```python
from build123d import *

# Parameters (mm, degrees)
SHELL1_T            = -1
SKETCH2_R           = 45
SKETCH2_R_2         = 3.125
SKETCH2_R_3         = 28.999861121
BOSS_EXTRUDE1_DEPTH = 2


with BuildPart() as part:
    # Sketch1 → Revolve1 (revolve)
    with BuildSketch(Plane(origin=(0, 0, 0), x_dir=(0, 0, -1), z_dir=(1, 0, 0))):
        with BuildLine():
            Line((0, 0), (-50.959835356, 0))
            Line((-50.959835356, 0), (-60.054255014, 0))
            Line((-60.054255014, 0), (-60.054255014, 30))
            Line((-60.054255014, 30), (-30.054255014, 29.5))
            ThreePointArc((-30.054255014, 29.5), (-27.754838856, 29.797720054), (-25.637373582, 30.742332522))
            ThreePointArc((-25.637373582, 30.742332522), (-22.902920152, 32.314145749), (-20.042663952, 33.643343571))
            ThreePointArc((-20.042663952, 33.643343571), (-10.179122164, 36.1760026), (0, 35.877187771))
            Line((0, 35.877187771), (0, 34.862194457))
            Line((0, 34.862194457), (0, 0))
        make_face()
    revolve(axis=Axis((0, 0, 0), (0, 0, 1)))

    # Shell1
    shell1_openings = [part.faces().sort_by_distance(p)[0] for p in [
        (0, 0, 0),
        (0, 0, 60.054255014),
    ]]
    offset(amount=SHELL1_T, openings=shell1_openings, kind=Kind.INTERSECTION)

    # Sketch2 → Boss-Extrude1 (add)
    with BuildSketch(Plane.XY.offset(60.054255014)):
        Circle(SKETCH2_R)
        with Locations((0, 37.5)):
            Circle(SKETCH2_R_2, mode=Mode.SUBTRACT)
        with Locations((37.5, 0)):
            Circle(SKETCH2_R_2, mode=Mode.SUBTRACT)
        with Locations((0, -37.5)):
            Circle(SKETCH2_R_2, mode=Mode.SUBTRACT)
        with Locations((-37.5, 0)):
            Circle(SKETCH2_R_2, mode=Mode.SUBTRACT)
        Circle(SKETCH2_R_3, mode=Mode.SUBTRACT)
    extrude(amount=-BOSS_EXTRUDE1_DEPTH)


solid = part.part
```
Work out the finished part from the listing and answer in its coordinate system (mm). A direction names the side the tool comes from. Give positions to 0.01 mm unless a question says otherwise; leave off trailing zeros. Loops run counter-clockwise (first coordinate to the right, second up) from the corner with the lowest first, then second, coordinate; pieces in that order, holes last. Notation, with made-up numbers: (38.5, 34) -> (74.5, 34) arc R15 cw to (74.5, 42) -> close; hole circle Ø4 at (-40, 86.5). An arc over 180 degrees is marked (long way). Put each result on its own line as item: value. Start each with the question number.
Item 1: The mould has two halves that part along Z. Classify faces 4 (the face through (29.023, -6.445, 43.858)), 5 (the face through (17.492, -22.812, 44.853)), 6 (the face through (-0.4, -34.4, 59.1)): released by +Z, released by -Z, zero draft, split by the parting line, or undercut.
Item 2: Find the intervals of material crossed by L1, parallel to Y at x = 0, z = 59 (3 decimals); L2, parallel to Z at x = 7, y = 37.5; L3, parallel to Y at x = 10.5, z = 6, in increasing order. Write a range as [from, to].
Item 3: Each of these flat-tipped pins is pushed along its axis until it touches: P1, Ø8, axis at y = -31, z = 31, coming from the +X side; P2, Ø6, axis at y = 15.5, z = 34, coming from the +X side; P3, Ø4, axis at y = -22.5, z = 26.5, coming from the -X side; P4, Ø3, axis at x = 25, y = -0.5, coming from the +Z side (1 decimal). Where does it stop, or does it pass through?
Item 4: The part is cut by section A-A (z = 35). Give the vertices of the cut face in (x, y), then the cut area to 3 significant figures.
Item 5: Which of the six approach directions +Z, -Z, +X, -X, +Y, -Y give full straight-line access (tool end or side, diameter ignored) to faces 1 (the face through (-21, 21, 60.054)), 2 (the face through (-1, 31, 58.054)), 3 (the face through (-0.4, 40.6, 59.1))?
Item 6: The part is cut by section B-B (y = 0). State how many separate pieces and enclosed holes the cut face has, then the cut area to 3 significant figures.
Answers below:
1. face 4: undercut
1. face 5: released by +Z
1. face 6: zero draft
2. L1: [-45, -40.625], [-34.375, -28.982], [28.982, 34.375], [40.625, 45]
2. L2: [58.05, 60.05]
2. L3: [-34.85, -33.81], [33.81, 34.85]
3. P1: x = 11.93
3. P2: x = 26.79
3. P3: x = -22.84
3. P4: through
4. outline: circle Ø59.16 at (0, 0); hole circle Ø57.16 at (0, 0)
4. area: 183 mm2
5. face 1: +Z, +X, -X, +Y, -Y
5. face 2: none
5. face 3: +Z
6. separate pieces: 4
6. enclosed holes: 0
6. area: 158 mm2
